```python
from build123d import *

# Parameters (mm, degrees)
SKETCH1_W           = 250
SKETCH1_H           = 250
SKETCH1_W_2         = 230
SKETCH1_H_2         = 230
BOSS_EXTRUDE1_DEPTH = 90
SKETCH2_W           = 200
SKETCH2_H           = 70
CUT_EXTRUDE1_DEPTH  = 50
FILLET1_R           = 20
SKETCH3_W           = 210
SKETCH3_H           = 90
CUT_EXTRUDE2_DEPTH  = 251
SKETCH4_R           = 2.5
CUT_EXTRUDE3_DEPTH  = 10


with BuildPart() as part:
    # Sketch1 → Boss-Extrude1 (new body)
    with BuildSketch(Plane(origin=(0, 0, 0), x_dir=(1, 0, 0), z_dir=(0, 1, 0))):
        Rectangle(SKETCH1_W, SKETCH1_H)
        Rectangle(SKETCH1_W_2, SKETCH1_H_2, mode=Mode.SUBTRACT)
    extrude(amount=BOSS_EXTRUDE1_DEPTH)

    # Sketch2 → Cut-Extrude1 (cut)
    with BuildSketch(Plane.XY.offset(125)):
        with Locations((0, 35)):
            Rectangle(SKETCH2_W, SKETCH2_H)
    extrude(amount=-CUT_EXTRUDE1_DEPTH, mode=Mode.SUBTRACT)

    # Fillet1
    fillet1_edges = [part.edges().sort_by_distance(p)[0] for p in [
        (-115, 45, 115),
        (115, 45, 115),
        (115, 45, -115),
        (-115, 45, -115),
        (-125, 45, 125),
        (125, 45, 125),
        (125, 45, -125),
        (-125, 45, -125),
    ]]
    fillet(fillet1_edges, radius=FILLET1_R)

    # Sketch3 → Cut-Extrude2 (cut, through all)
    with BuildSketch(Plane.ZY.offset(125)):
        with Locations((20, 45)):
            Rectangle(SKETCH3_W, SKETCH3_H)
    extrude(amount=-CUT_EXTRUDE2_DEPTH, mode=Mode.SUBTRACT)

    # Sketch4 → Cut-Extrude3 (cut)
    with BuildSketch(Plane(origin=(0, 0, -125), x_dir=(-1, 0, 0), z_dir=(0, 0, -1))):
        with Locations((85, 70)):
            Circle(SKETCH4_R)
        with Locations((-85, 70)):
            Circle(SKETCH4_R)
    extrude(amount=-CUT_EXTRUDE3_DEPTH, mode=Mode.SUBTRACT)


solid = part.part
```
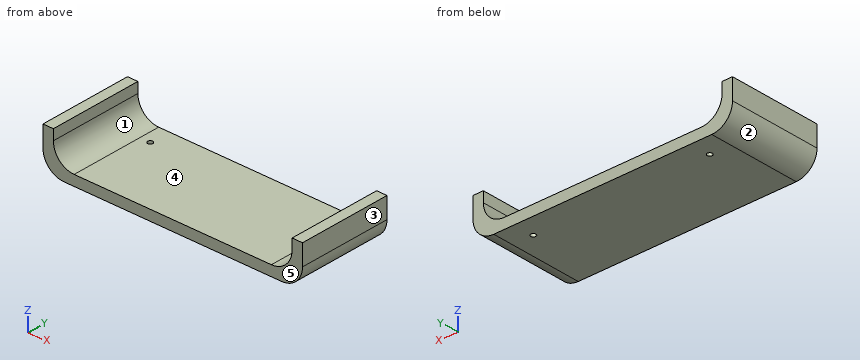
The listing builds one solid part. Answer for the finished solid, in the listing's coordinates (mm). Face numbers are marked on the shaded views. A direction names the side the tool comes from. Give positions to 0.01 mm unless a question says otherwise; leave off trailing zeros. Write each loop counter-clockwise with the first axis right and the second up, starting at its lowest first coordinate (ties: lowest second). Pieces come first, ordered by that corner, then holes. Notation, with made-up numbers: (13, 83) -> (62, 83) arc R25 ccw to (62, 112) -> close; hole circle Ø1 at (51.5, 53.25). An arc over 180 degrees is marked (long way). Write item = value, one per line. Start each with the question number.
1) Determine the mould class of the marked faces 1, 2 and 3 for opening direction X: +X half, -X half, draft (parallel to the pull), parting line (faces both ways), or undercut.
2) The part is cut by section C-C, the plane z = -90.5. Determine the outline of the cut face in (x, y), and give its area (3 significant figures).
3) The part is cut by section B-B, the plane y = 70. Determine the outline of the cut face in (x, z).
4) The part is cut by section D-D, the plane y = 40.5. Determine the outline of the cut face in (x, z), and give its area (3 significant figures).
5) Each of these flat-tipped pins is pushed along its axis until it touches: pin 1 (8 mm diameter, centred on x = -85, y = 70, fed in from +Z); pin 2 (5 mm diameter, centred on y = 66, z = -121, fed in from -X); pin 3 (5 mm diameter, centred on x = -63, z = -113, fed in from +Y). Where does it stop, or does it pass through?
6) Which of the six approach directions +Z, -Z, +X, -X, +Y, -Y give full straight-line access (tool end or side, diameter ignored) to the marked faces 4 and 5?
7) The part is cut by section A-A, the plane x = -85. Determine the outline of the cut face in (y, z).
8) Straight lines are drawn through the part: line 1 along X through (y, z) = (47, -90); line 2 along Y through (x, z) = (85, -119.25); line 3 along Z through (x, y) = (-55, 36). For each, find the intervals that lie inside material, in ascending order.
Solutions:
q1.face_1 = undercut
q1.face_2 = -X half
q1.face_3 = +X half
q2.outline = (-125, 0) -> (-115, 0) -> (-115, 90) -> (-125, 90) -> close; (115, 0) -> (125, 0) -> (125, 90) -> (115, 90) -> close
q2.area = 1,800 mm²
q3.outline = (-125, -105) arc R20 ccw to (-105, -125) -> (-87.5, -125) -> (-87.5, -115) -> (-95, -115) arc R20 cw to (-115, -95) -> (-115, -85) -> (-125, -85) -> close; (-82.5, -125) -> (82.5, -125) -> (82.5, -115) -> (-82.5, -115) -> close; (87.5, -125) -> (105, -125) arc R20 ccw to (125, -105) -> (125, -85) -> (115, -85) -> (115, -95) arc R20 cw to (95, -115) -> (87.5, -115) -> close
q4.outline = (-125, -105) arc R20 ccw to (-105, -125) -> (105, -125) arc R20 ccw to (125, -105) -> (125, -85) -> (115, -85) -> (115, -95) arc R20 cw to (95, -115) -> (-95, -115) arc R20 cw to (-115, -95) -> (-115, -85) -> (-125, -85) -> close
q4.area = 3,100 mm²
q5.pin_1 = -115
q5.pin_2 = -119.76
q5.pin_3 = 90
q6.face_4 = +Z, +Y, -Y
q6.face_5 = +Z, -Z, +X, -X, -Y
q7.outline = (0, -125) -> (67.5, -125) -> (67.5, -115) -> (0, -115) -> close; (72.5, -125) -> (90, -125) -> (90, -115) -> (72.5, -115) -> close
q8.line_1 = -125 to -115, 115 to 125
q8.line_2 = 0 to 67.5, 72.5 to 90
q8.line_3 = -125 to -115
